The model under review builds one solid part; all positions refer to its coordinate system, in mm. A direction names the side the tool comes from. Coordinates: 2 decimals unless noted, no trailing zeros. Order: outer loops, then holes, each group sorted by start corner. A loop starts at its lowest first (then second) coordinate and runs counter-clockwise, first axis right, second up. Notation, with made-up numbers: (31, 12) -> (52, 12) arc R11 ccw to (52, 22) -> close; hole circle Ø2 at (35, 22.5). An arc over 180 degrees is marked (long way). Use one line per item in the form item = value.
from build123d import *

# Parameters (mm, degrees)
SKETCH2_W           = 19.05
SKETCH2_H           = 19.05
SKETCH2_W_2         = 15.875
SKETCH2_H_2         = 15.875
BOSS_EXTRUDE1_DEPTH = 457.2
FILLET1_R           = 1.905
FILLET2_R           = 0.3175


with BuildPart() as part:
    # Sketch2 → Boss-Extrude1 (new, symmetric)
    with BuildSketch(Plane.XY):
        Rectangle(SKETCH2_W, SKETCH2_H)
        Rectangle(SKETCH2_W_2, SKETCH2_H_2, mode=Mode.SUBTRACT)
    extrude(amount=BOSS_EXTRUDE1_DEPTH, both=True)

    # Fillet1
    fillet1_edges = [part.edges().sort_by_distance(p)[0] for p in [
        (-9.525, -9.525, 0),
        (-9.525, 9.525, 0),
        (9.525, 9.525, 0),
        (9.525, -9.525, 0),
    ]]
    fillet(fillet1_edges, radius=FILLET1_R)

    # Fillet2
    fillet2_edges = [part.edges().sort_by_distance(p)[0] for p in [
        (-7.9375, -7.9375, 0),
        (7.9375, -7.9375, 0),
        (7.9375, 7.9375, 0),
        (-7.9375, 7.9375, 0),
    ]]
    fillet(fillet2_edges, radius=FILLET2_R)


solid = part.part
Item 1: Draft analysis for pull direction X (two halves, no side actions). For faces 1 (the face through (-9.525, 0, 6)), 2 (the face through (0, -7.938, 6)), 3 (the face through (0, 9.525, 6)), state which applies: released by +X, released by -X, zero draft, split by the parting line, or undercut.
Results found:
face_1 = released by -X
face_2 = undercut
face_3 = zero draft
Item 2: We need section B-B (z = 24.5). Write out the cut boundary in (x, y) (1 decimal), plus the area to 3 significant figures.
Results found:
outline = (-9.5, -7.6) arc R1.9 ccw to (-7.6, -9.5) -> (7.6, -9.5) arc R1.9 ccw to (9.5, -7.6) -> (9.5, 7.6) arc R1.9 ccw to (7.6, 9.5) -> (-7.6, 9.5) arc R1.9 ccw to (-9.5, 7.6) -> close; hole (-7.9, -7.6) arc R0.3 ccw to (-7.6, -7.9) -> (7.6, -7.9) arc R0.3 ccw to (7.9, -7.6) -> (7.9, 7.6) arc R0.3 ccw to (7.6, 7.9) -> (-7.6, 7.9) arc R0.3 ccw to (-7.9, 7.6) -> close
area = 108 mm²
Item 3: We need section A-A (x = 0). Write out the cut boundary in (y, z) (1 decimal), plus the area to 3 significant figures.
Results found:
outline = (-9.5, -457.2) -> (-7.9, -457.2) -> (-7.9, 457.2) -> (-9.5, 457.2) -> close; (7.9, -457.2) -> (9.5, -457.2) -> (9.5, 457.2) -> (7.9, 457.2) -> close
area = 2,900 mm²
Item 4: Tool access review of faces 4 (the face through (0, -9.525, 6)), 5 (the face through (7.938, 0, 6)): name each direction out of +Z, -Z, +X, -X, +Y, -Y from which nothing blocks a thin tool from reaching the whole face with its end or side.
Results found:
face_4 = +Z, -Z, +X, -X, -Y
face_5 = +Z, -Z
Item 5: To check wall thickness, follow L1, parallel to Y at x = 4.25, z = -416.5 (1 decimal); L2, parallel to Y at x = 8, z = 183.5. State the ranges of each line that lie inside material, in increasing order. Write a range as from..to.
Results found:
L1 = -9.5..-7.9, 7.9..9.5
L2 = -9.49..9.49
